Verification items for the finished model (mm, model axes). A direction names the side the tool comes from. Give positions to 0.01 mm unless a question says otherwise; leave off trailing zeros. Order: outer loops, then holes, each group sorted by start corner. A loop starts at its lowest first (then second) coordinate and runs counter-clockwise, first axis right, second up.
Solid Edge part; units mm, degrees
sketch "Sketch1" plane through (0, 0, 0) normal (0, -1, 0) x (1, 0, 0)
  line L0 (33, 0) -> (33, 90)
  line L1 (33, 90) -> (13, 90)
  line L2 (13, 90) -> (13, 72)
  arc A0 (-13, 72) -> (13, 72) centre (0, 72) ccw
  line L3 (-13, 90) -> (-13, 72)
  line L4 (-33, 90) -> (-13, 90)
  line L5 (-33, 0) -> (-33, 90)
  line L6 (0, 0) -> (-33, 0)
  line L7 (0, 0) -> (33, 0)
extrude "Protrusion1" add sketch "Sketch1" against normal blind 20
sketch "Sketch2" plane through (0, 0, 0) normal (0, 0, 1) x (1, 0, 0)
  line L0 (33, 0) -> (33, -25)
  line L1 (33, -25) -> (20, -25)
  arc A0 (-20, -25) -> (20, -25) centre (0, -25) ccw
  line L2 (-33, -25) -> (-20, -25)
  line L3 (-33, 0) -> (-33, -25)
extrude "ExtrudedProtrusion_2" add sketch "Sketch2" along normal blind 35 material side at (32.95, -12.5, 0)
(1) Section check C-C, the plane z = 14. Enter the section's corners in (x, y).
Solved:
outline: (-33, -25) - (-20, -25) arc R20 ccw to (20, -25) - (33, -25) - (33, 20) - (-33, 20) - close
(2) Go/stop test with flat-tipped pins: pin 1 (6 mm diameter, centred on x = -8.5, y = -29, fed in from -Z); pin 2 (5 mm diameter, centred on x = 4, y = 5.5, fed in from +Z); pin 3 (22.5 mm diameter, centred on x = 4, y = -19, fed in from +Z); pin 4 (6.5 mm diameter, centred on x = -28.5, z = 24.5, fed in from -Y). Record where each tip stops, or that it passes through.
Solved:
pin 1: stops at z = 0
pin 2: stops at z = 60.74
pin 3: stops at z = 35
pin 4: stops at y = -25
(3) Section check B-B, the plane x = 0. Enter the section's corners in (y, z).
Solved:
outline: (-45, 0) - (20, 0) - (20, 59) - (0, 59) - (0, 35) - (-45, 35) - close
(4) Release check for a two-part mould opening along X. For faces 1 (the flat face through (0, 0, 57)), 2 (the flat face through (33, 2, 34)), 3 (the flat face through (-13, 10, 81)) record: pulls with the +X half, pulls with the -X half, needs draft (parallel to the pull), parting line crosses it, or undercut.
Solved:
face 1: needs draft
face 2: pulls with the +X half
face 3: undercut
(5) Set-up check for faces 4 (the flat face through (-27, -25, 17)), 5 (the flat face through (0, -17, 35)), 6 (the flat face through (13, 10, 81)), 7 (the flat face through (27, -25, 17)): record each of +Z, -Z, +X, -X, +Y, -Y from which the full face is reachable in a straight line by a thin tool's end or side.
Solved:
face 4: +Z, -Z, -X, -Y
face 5: +Z, +X, -X, -Y
face 6: +Z, +Y, -Y
face 7: +Z, -Z, +X, -Y
(6) Section check A-A, the plane z = 77.5. Enter the section's corners in (x, y), then the cut area to 3 significant figures.
Solved:
outline: (-33, 0) - (-13, 0) - (-13, 20) - (-33, 20) - close; (13, 0) - (33, 0) - (33, 20) - (13, 20) - close
area: 800 mm2
(7) Scan lines: line 1 (X direction, y = 11, z = 83); line 2 (Y direction, x = -29.5, z = 48.5); line 3 (Z direction, x = -10, y = -20.5). Record each from-to range of solid material in increasing order.
Solved:
line 1: x = -33 to -13, 13 to 33
line 2: y = 0 to 20
line 3: z = 0 to 35
(8) Section check D-D, the plane y = -6. Enter the section's corners in (x, z), then the cut area to 3 significant figures.
Solved:
outline: (-33, 0) - (33, 0) - (33, 35) - (-33, 35) - close
area: 2,310 mm2
